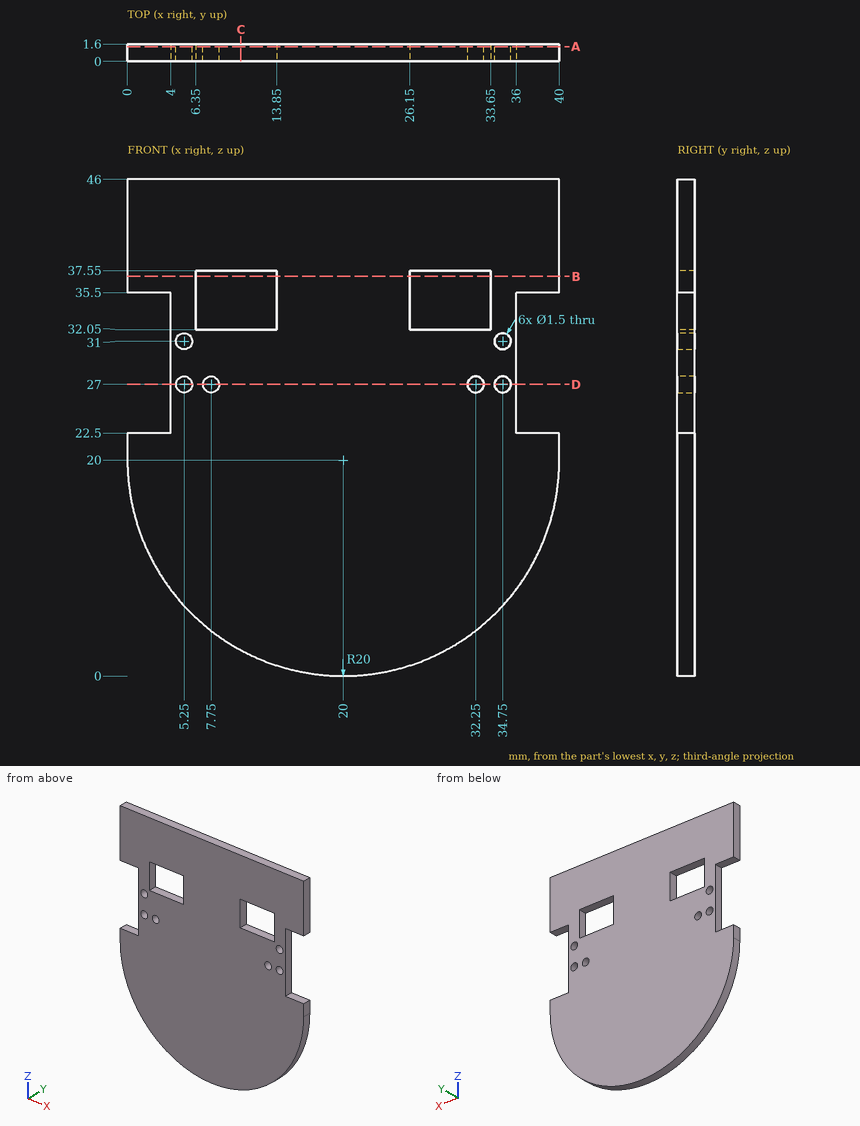
Can you work these out from the drawing? Everything is in mm from the part's minimum corner. Give positions to 0.01 mm unless a question says otherwise; leave off trailing zeros. Order: outer loops, then holes, each group sorted by start corner. A loop starts at its lowest first (then second) coordinate and runs counter-clockwise, first axis right, second up.
1. Suppose I cut it at C-C (x = 10.5). List the corners of the cut face in (y, z) for me.
2. Suppose I cut it at B-B (z = 37). List the corners of the cut face in (x, y) for me.
3. Suppose I cut it at D-D (z = 27). List the corners of the cut face in (x, y) for me, plus the area to 3 significant figures.
4. Suppose I cut it at A-A (y = 1.35). Give the number of separate pieces and of enclosed holes in the cut face, plus the area to 3 significant figures.
5. I need wall thicknesses on L1, parallel to X at y = 1.35, z = 27; L2, parallel to X at y = 0.7, z = 31; L3, parallel to Z at x = 5.25, y = 1. Which ranges of each line are inside material? Lowest first, please.
6. Will these pins go through, and if not, where does the flat tip stop? P1, Ø5, axis at x = 4.5, z = 38.5, coming from the -Y side; P2, Ø0.5, axis at y = 0.5, z = 34.5, coming from the +X side; P3, Ø1.4, axis at x = 7.75, z = 27, coming from the +Y side.
Solved:
1. outline: (0, 2.4) - (1.6, 2.4) - (1.6, 32.05) - (0, 32.05) - close; (0, 37.55) - (1.6, 37.55) - (1.6, 46) - (0, 46) - close
2. outline: (0, 0) - (6.35, 0) - (6.35, 1.6) - (0, 1.6) - close; (13.85, 0) - (26.15, 0) - (26.15, 1.6) - (13.85, 1.6) - close; (33.65, 0) - (40, 0) - (40, 1.6) - (33.65, 1.6) - close
3. outline: (4, 0) - (4.5, 0) - (4.5, 1.6) - (4, 1.6) - close; (6, 0) - (7, 0) - (7, 1.6) - (6, 1.6) - close; (8.5, 0) - (31.5, 0) - (31.5, 1.6) - (8.5, 1.6) - close; (33, 0) - (34, 0) - (34, 1.6) - (33, 1.6) - close; (35.5, 0) - (36, 0) - (36, 1.6) - (35.5, 1.6) - close
3. area: 41.6 mm2
4. separate pieces: 1
4. enclosed holes: 8
4. area: 1,470 mm2
5. L1: x = 4 to 4.5, 6 to 7, 8.5 to 31.5, 33 to 34, 35.5 to 36
5. L2: x = 4 to 4.5, 6 to 34, 35.5 to 36
5. L3: z = 6.49 to 26.25, 27.75 to 30.25, 31.75 to 46
6. P1: stops at y = 0
6. P2: stops at x = 36
6. P3: passes through
